from build123d import *

# Parameters (mm, degrees)
F1_DEPTH = 2.54
F2_R     = 1.27
F3_R     = 0.254
F4_R     = 1.27
F5_R     = 0.254
F6_R     = 1.27
F7_R     = 1.27


with BuildPart() as f1:
    # F0 (on Right) → F1 (new body)
    with BuildSketch(Plane.YZ):
        Polygon((-29.258431, 13.248995), (-30.3611, 12.618899), (-27.350505, 12.242574), (-23.780038, -2.022478), (-24.11806, -2.703207), (-23.618102, -3.27826), (-22.994532, -2.022478), (-26.738045, 12.933947), align=None)
    extrude(amount=F1_DEPTH)

    # F2
    f2_edges = [f1.edges().sort_by_distance(p)[0] for p in [
        (1.27, -22.994532, -2.022478),
    ]]
    fillet(f2_edges, radius=F2_R)

    # F3
    f3_edges = [f1.edges().sort_by_distance(p)[0] for p in [
        (1.27, -23.618102, -3.27826),
    ]]
    fillet(f3_edges, radius=F3_R)

    # F4
    f4_edges = [f1.edges().sort_by_distance(p)[0] for p in [
        (1.27, -23.780038, -2.022478),
    ]]
    fillet(f4_edges, radius=F4_R)

    # F5
    f5_edges = [f1.edges().sort_by_distance(p)[0] for p in [
        (1.27, -24.11806, -2.703207),
    ]]
    fillet(f5_edges, radius=F5_R)

    # F6
    f6_edges = [f1.edges().sort_by_distance(p)[0] for p in [
        (1.27, -26.738045, 12.933947),
    ]]
    fillet(f6_edges, radius=F6_R)

    # F7
    f7_edges = [f1.edges().sort_by_distance(p)[0] for p in [
        (1.27, -27.350505, 12.242574),
    ]]
    fillet(f7_edges, radius=F7_R)


solid = f1.part
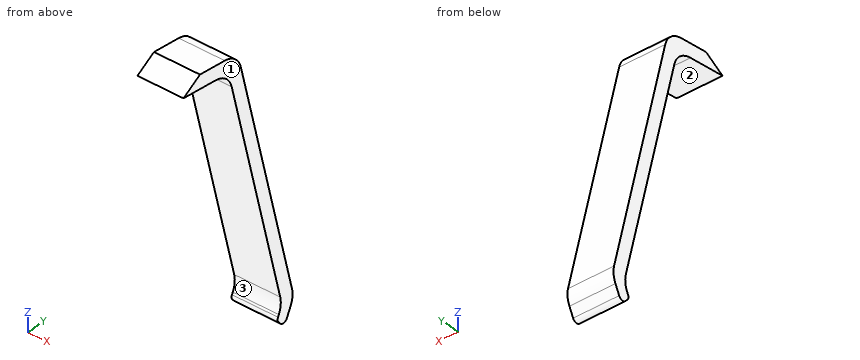
Could you check a few things on this model? Use its own coordinates, in mm. Face numbers are marked on the shaded views. Coordinates: 2 decimals unless noted, no trailing zeros. Order: outer loops, then holes, each group sorted by start corner. A loop starts at its lowest first (then second) coordinate and runs counter-clockwise, first axis right, second up.
Q1. Thinking about a two-plate mould opening in Z: for the marked faces 1, 2 and 3, which applies, released by +Z, released by -Z, zero draft, split by the parting line, or undercut?
Q2. Will this pin go through, and if not, where does the flat tip stop? pin 1 (2 mm diameter, centred on y = -25, z = 8, fed in from -X).
Q3. Suppose I cut it at A-A on x = 2. Please give me the cut outline in (y, z), and give its area (3 significant figures).
Q4. Please list where these lines run through material, in increasing order: L1, parallel to Z at x = 1.4, y = -28; L2, parallel to Y at x = 0.25, z = 4.25; L3, parallel to Z at x = 0.35, y = -29.25.
Q5. Suppose I cut it at C-C on z = 9.75. Please give me the cut outline in (x, y).
Q6. Suppose I cut it at B-B on y = -29.5. Please give me the cut outline in (x, z).
Answer:
1. face 1: zero draft
1. face 2: released by -Z
1. face 3: undercut
2. pin 1: stops at x = 0
3. outline: (-30.36, 12.62) - (-28.21, 12.35) arc R1.27 cw to (-27.14, 11.4) - (-23.89, -1.57) arc R1.27 cw to (-23.99, -2.44) - (-24.04, -2.55) arc R0.25 ccw to (-24.01, -2.83) - (-23.87, -2.99) arc R0.25 ccw to (-23.45, -2.94) - (-23.2, -2.44) arc R1.27 ccw to (-23.11, -1.57) - (-26.53, 12.09) arc R1.27 ccw to (-27.6, 13.04) - (-29.26, 13.25) - close
3. area: 14.3 mm2
4. L1: z = 12.3 to 13.09
4. L2: y = -25.35 to -24.56
4. L3: z = 12.48 to 13.25
5. outline: (0, -26.73) - (2.54, -26.73) - (2.54, -25.94) - (0, -25.94) - close
6. outline: (0, 12.51) - (2.54, 12.51) - (2.54, 13.11) - (0, 13.11) - close
